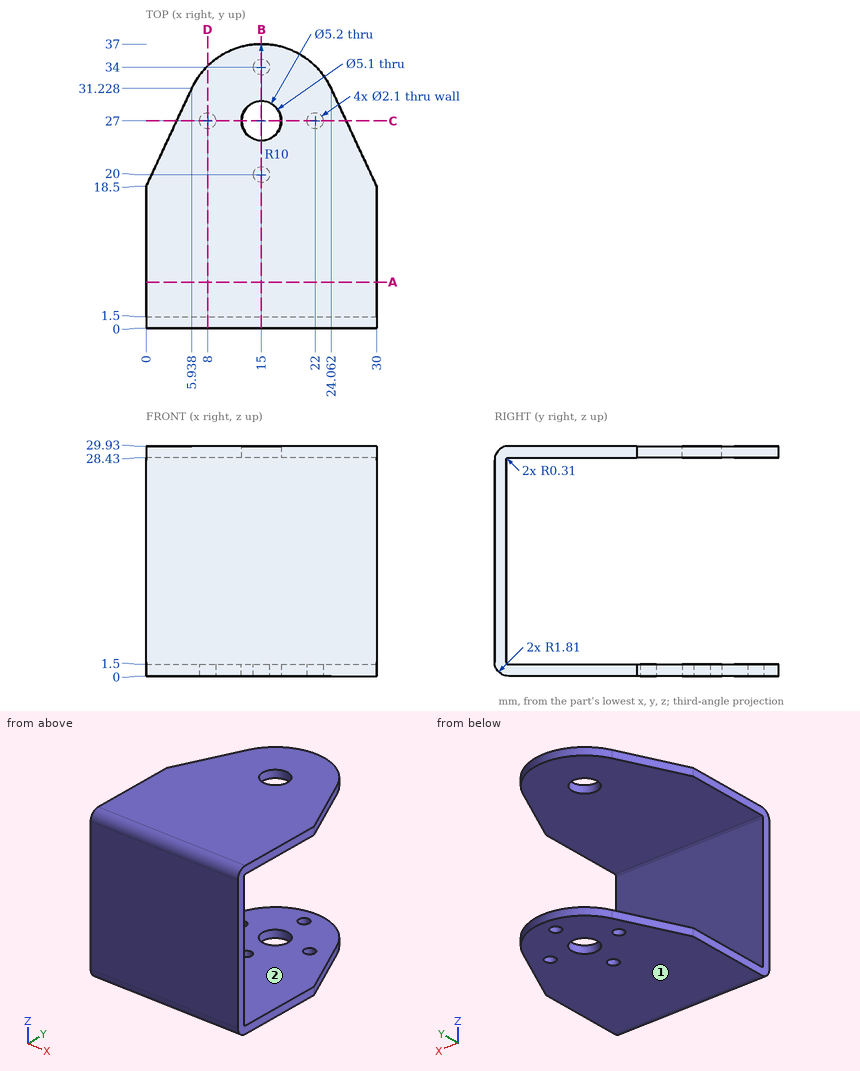
Here's the drawing with two shaded views (mm, measured from the low corner). I have some questions. A direction names the side the tool comes from. Give positions to 0.01 mm unless a question says otherwise; leave off trailing zeros. Order: outer loops, then holes, each group sorted by start corner. A loop starts at its lowest first (then second) coordinate and runs counter-clockwise, first axis right, second up. Notation, with made-up numbers: (68.5, -21) -> (79.5, -21) arc R16 ccw to (79.5, 10) -> close; hole circle Ø9 at (46.5, -21). An arc over 180 degrees is marked (long way). Use a Markdown table: item, result. Add a question column.
Item 1: Imagine slicing it at D-D on x = 8. Please give me the cut outline in (y, z).
Item 2: Imagine slicing it at A-A on y = 6. Please give me the cut outline in (x, z).
Item 3: Imagine slicing it at B-B on x = 15. Please give me the cut outline in (y, z), plus the area to 3 significant figures.
Item 4: I need wall thicknesses on line 1 (Z direction, x = 10.5, y = 2.5); line 2 (Y direction, x = 26.5, z = 24.75). Which ranges of each line are inside material? Lowest first, please.
Item 5: Imagine slicing it at C-C on y = 27. Give the number of separate pieces and of enclosed holes in the cut face.
Item 6: Will these pins go through, and if not, where does the flat tip stop? pin 1 (3 mm diameter, centred on x = 21.5, y = 4, fed in from -Z); pin 2 (3 mm diameter, centred on y = 21.5, z = 25, fed in from -X); pin 3 (8 mm diameter, centred on x = 8, z = 21, fed in from +Y).
Item 7: For the marked faces 1 and 2, which set-ups out of +Z, -Z, +X, -X, +Y, -Y let a thin tool reach every point of the face, with its end or its side?
Data:
| question | item | result |
|---|---|---|
| 1 | outline | (0, 1.81) arc R1.81 ccw to (1.81, 0) -> (25.95, 0) -> (25.95, 1.5) -> (1.81, 1.5) arc R0.31 cw to (1.5, 1.81) -> (1.5, 28.12) arc R0.31 cw to (1.81, 28.43) -> (34.14, 28.43) -> (34.14, 29.93) -> (1.81, 29.93) arc R1.81 ccw to (0, 28.12) -> close; (28.05, 0) -> (34.14, 0) -> (34.14, 1.5) -> (28.05, 1.5) -> close |
| 2 | outline | (0, 0) -> (30, 0) -> (30, 1.5) -> (0, 1.5) -> close; (0, 28.43) -> (30, 28.43) -> (30, 29.93) -> (0, 29.93) -> close |
| 3 | outline | (0, 1.81) arc R1.81 ccw to (1.81, 0) -> (18.95, 0) -> (18.95, 1.5) -> (1.81, 1.5) arc R0.31 cw to (1.5, 1.81) -> (1.5, 28.12) arc R0.31 cw to (1.81, 28.43) -> (24.45, 28.43) -> (24.45, 29.93) -> (1.81, 29.93) arc R1.81 ccw to (0, 28.12) -> close; (21.05, 0) -> (24.4, 0) -> (24.4, 1.5) -> (21.05, 1.5) -> close; (29.55, 28.43) -> (37, 28.43) -> (37, 29.93) -> (29.55, 29.93) -> close; (29.6, 0) -> (32.95, 0) -> (32.95, 1.5) -> (29.6, 1.5) -> close; (35.05, 0) -> (37, 0) -> (37, 1.5) -> (35.05, 1.5) -> close |
| 3 | area | 128 mm² |
| 4 | line 1 | z = 0 to 1.5, 28.43 to 29.93 |
| 4 | line 2 | y = 0 to 1.5 |
| 5 | separate pieces | 6 |
| 5 | enclosed holes | 0 |
| 6 | pin 1 | stops at z = 0 |
| 6 | pin 2 | passes through |
| 6 | pin 3 | stops at y = 1.5 |
| 7 | face 1 | -Z, +X, -X, +Y, -Y |
| 7 | face 2 | +X, -X, +Y |
